Can you work these out from the drawing? Everything is in mm from the part's minimum corner. Coordinates: 2 decimals unless noted, no trailing zeros. Order: outer loops, then holes, each group sorted by start corner. A loop starts at its lowest first (then second) coordinate and runs counter-clockwise, first axis right, second up. Notation, with made-up numbers: (-21, 4) -> (28, 4) arc R18 cw to (28, 16) -> close; hole circle Ø1 at (-8, 35.5). An arc over 180 degrees is marked (long way). Return JSON: item names as keys, results as strings. Group by question number.
1) If we section it at B-B, the plane y = 10: Please give me the cut outline in (x, z).
2) If I drill on probe 1 along Y at (x, z) = (18.75, 191); probe 2 along X at (y, z) = (11.25, 161.5), over which ranges is the centre line in solid material (lowest first)? Write a range as from..to.
3) For pin 1 (1.5 mm diameter, centred on y = 3, z = 125.5, fed in from -X); pin 2 (2.5 mm diameter, centred on x = 9.5, z = 175, fed in from -Y); pin 3 (2 mm diameter, centred on x = 9, z = 106, fed in from +Y); pin 4 (2.5 mm diameter, centred on y = 9, z = 174.5, fed in from -X), each with a flat end and sliding along its axis, tell me the tip position at first contact or that it passes through.
4) If we section it at A-A, the plane z = 173: Please give me the cut outline in (x, y), then the cut area to 3 significant figures.
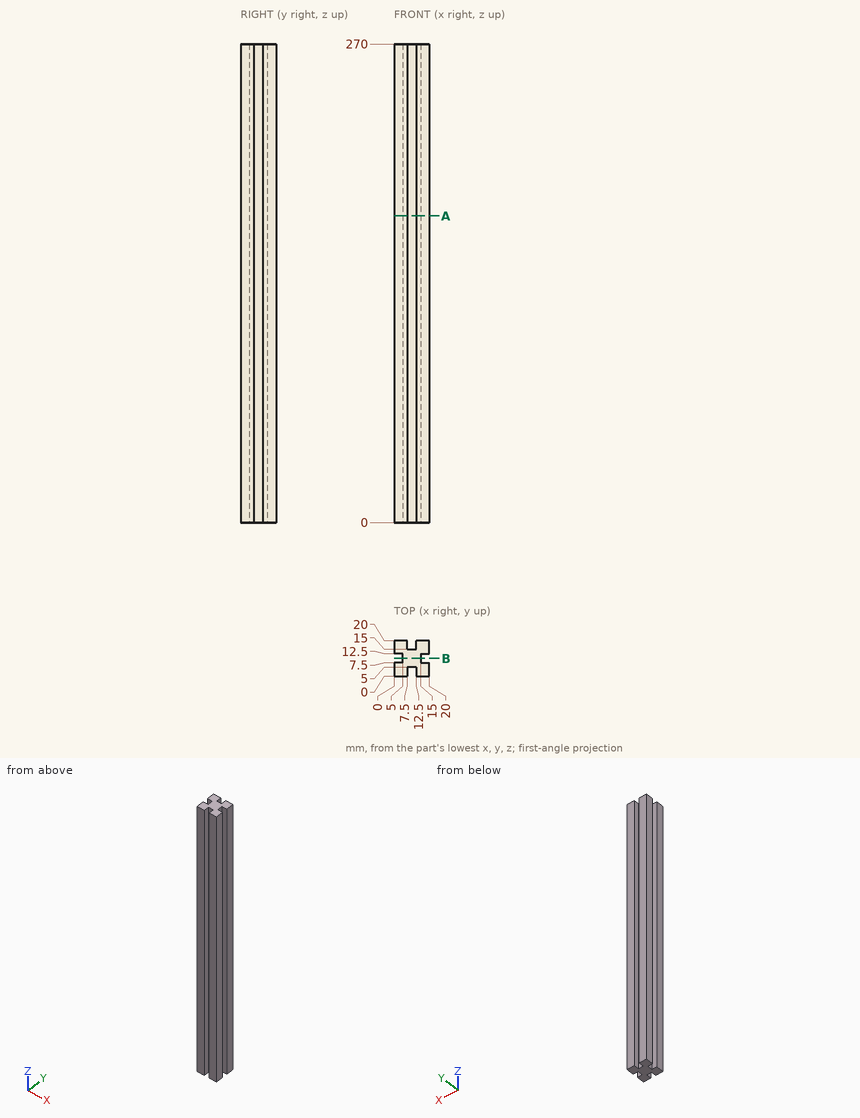
Result sheet:
{
 "1": {"outline": "(5, 0) -> (15, 0) -> (15, 270) -> (5, 270) -> close"},
 "2": {"probe 1": "y = 0..7.5, 12.5..20", "probe 2": "x = 5..15"},
 "3": {"pin 1": "stops at x = 0", "pin 2": "stops at y = 5", "pin 3": "stops at y = 15", "pin 4": "stops at x = 5"},
 "4": {"outline": "(0, 0) -> (7.5, 0) -> (7.5, 5) -> (12.5, 5) -> (12.5, 0) -> (20, 0) -> (20, 7.5) -> (15, 7.5) -> (15, 12.5) -> (20, 12.5) -> (20, 20) -> (12.5, 20) -> (12.5, 15) -> (7.5, 15) -> (7.5, 20) -> (0, 20) -> (0, 12.5) -> (5, 12.5) -> (5, 7.5) -> (0, 7.5) -> close", "area": "300 mm2"}
}
